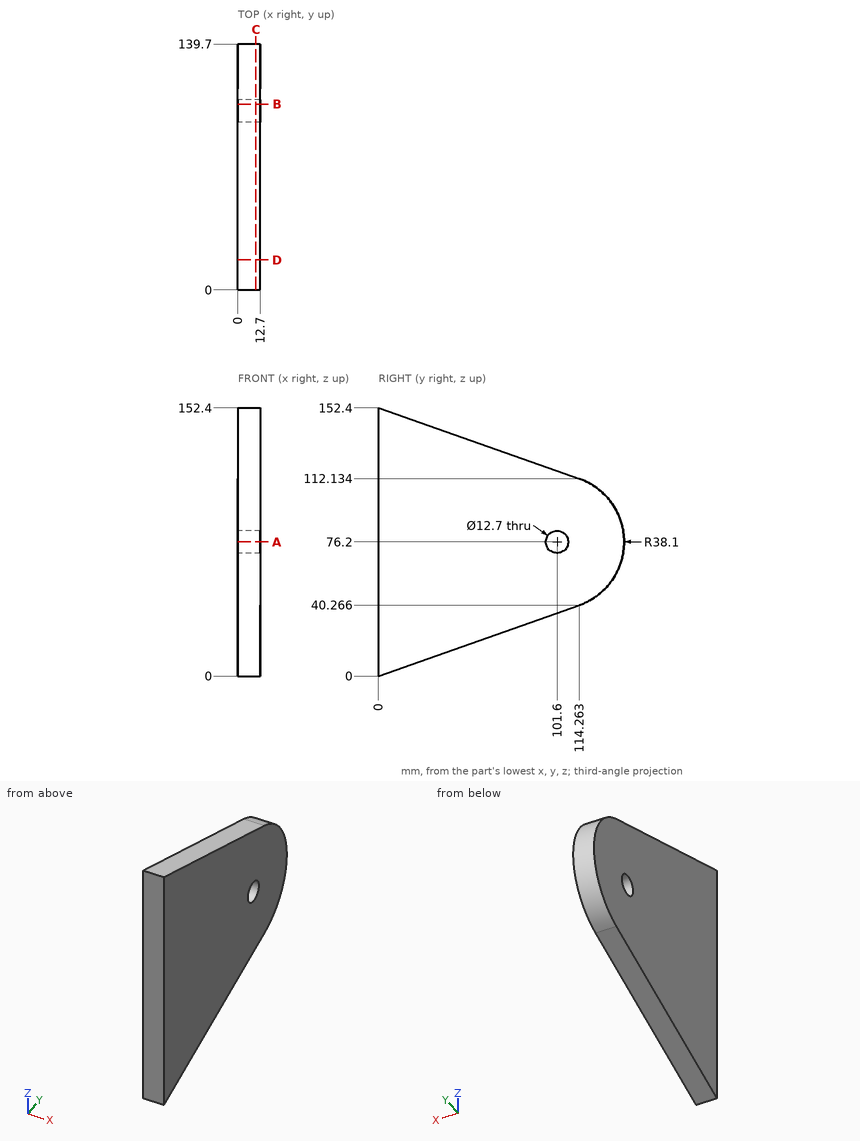
Geometry check sheet. Reference: drawing and pictorial views, mm from the part's lowest x, y, z. Give positions to 0.01 mm unless a question says otherwise; leave off trailing zeros. Write each loop counter-clockwise with the first axis right and the second up, starting at its lowest first coordinate (ties: lowest second). Pieces come first, ordered by that corner, then holes.
Item 1: Gauge pin test, flat ends, axial feed: pin 1 (1.5 mm diameter, centred on x = 9, y = 117.5, fed in from -Z); pin 2 (1 mm diameter, centred on x = 5.5, y = 79, fed in from +Z); pin 3 (11.5 mm diameter, centred on y = 101.6, z = 76.2, fed in from -X); pin 4 (4 mm diameter, centred on x = 2, z = 45.5, fed in from +Y). Record the tip position at first contact, or that the pin passes through.
Item 2: Scan lines: L1, parallel to Y at x = 7.5, z = 76.2; L2, parallel to Z at x = 10, y = 101.6; L3, parallel to Y at x = 12, z = 80. Record each from-to range of solid material in increasing order.
Item 3: Cross-section at D-D (y = 17). Enter the section's corners in (x, z), and give its area (3 significant figures).
Item 4: Cross-section at B-B (y = 105.5). Enter the section's corners in (x, z).
Item 5: Cross-section at C-C (x = 10.25). Enter the section's corners in (y, z).
Item 6: Cross-section at A-A (z = 76.2). Enter the section's corners in (x, y).
Report:
1. pin 1: stops at z = 41.24
1. pin 2: stops at z = 124.74
1. pin 3: passes through
1. pin 4: stops at y = 126.66
2. L1: y = 0 to 95.25, 107.95 to 139.7
2. L2: z = 35.8 to 69.85, 82.55 to 116.6
2. L3: y = 0 to 96.51, 106.69 to 139.51
3. outline: (0, 5.99) - (12.7, 5.99) - (12.7, 146.41) - (0, 146.41) - close
3. area: 1,780 mm2
4. outline: (0, 37.18) - (12.7, 37.18) - (12.7, 71.19) - (0, 71.19) - close; (0, 81.21) - (12.7, 81.21) - (12.7, 115.22) - (0, 115.22) - close
5. outline: (0, 0) - (114.26, 40.27) arc R38.1 ccw to (114.26, 112.13) - (0, 152.4) - close; hole circle Ø12.7 at (101.6, 76.2)
6. outline: (0, 0) - (12.7, 0) - (12.7, 95.25) - (0, 95.25) - close; (0, 107.95) - (12.7, 107.95) - (12.7, 139.7) - (0, 139.7) - close
